```python
from build123d import *

# Parameters (mm, degrees)
SKETCH1_R           = 0.6
BOSS_EXTRUDE1_DEPTH = 6.62
SKETCH2_W           = 5.82
SKETCH2_H           = 1.74
SKETCH2_H_2         = 1.53
CUT_EXTRUDE1_DEPTH  = 14.92
SKETCH5_W           = 0.8
SKETCH5_H           = 1.53
CUT_EXTRUDE4_DEPTH  = 6.62
SKETCH4_W           = 7.64
SKETCH4_H           = 5.82
SKETCH4_W_2         = 3.88
SKETCH4_H_2         = 3.6
CUT_EXTRUDE3_DEPTH  = 7.4
CHAMFER1_SIZE       = 0.5
SKETCH11_W          = 0.34
SKETCH11_H          = 0.8
CUT_EXTRUDE5_DEPTH  = 0.9


with BuildPart() as part:
    # Sketch1 → Boss-Extrude1 (new body)
    with BuildSketch(Plane.XY):
        Polygon((3.76, 2.4), (3.76, 3.2), (11.38, 3.2), (11.38, -3.2), (3.76, -3.2), (3.76, -2.4), (-2.54, -2.4), (-2.54, 2.4), align=None)
        Circle(SKETCH1_R, mode=Mode.SUBTRACT)
    extrude(amount=BOSS_EXTRUDE1_DEPTH)

    # Sketch2 → Cut-Extrude1 (cut, through all)
    with BuildSketch(Plane(origin=(11.38, 0, 0), x_dir=(0, 0, -1), z_dir=(1, 0, 0))):
        with Locations((-2.91, 0)):
            Rectangle(SKETCH2_W, SKETCH2_H)
        with Locations((-2.91, 2.435)):
            Rectangle(SKETCH2_W, SKETCH2_H_2)
        with Locations((-2.91, -2.435)):
            Rectangle(SKETCH2_W, SKETCH2_H_2)
    extrude(amount=-CUT_EXTRUDE1_DEPTH, mode=Mode.SUBTRACT)

    # Sketch5 → Cut-Extrude4 (cut)
    with BuildSketch(Plane(origin=(11.38, 0, 0), x_dir=(0, 0, -1), z_dir=(1, 0, 0))):
        with Locations((-6.22, 2.435)):
            Rectangle(SKETCH5_W, SKETCH5_H)
        with Locations((-6.22, -2.435)):
            Rectangle(SKETCH5_W, SKETCH5_H)
    extrude(amount=-CUT_EXTRUDE4_DEPTH, mode=Mode.SUBTRACT)

    # Sketch4 → Cut-Extrude3 (cut, through all)
    with BuildSketch(Plane.XZ.offset(3.2)):
        with Locations((1.28, 2.91)):
            Rectangle(SKETCH4_W, SKETCH4_H)
        with Locations((8.24, 1.8)):
            Rectangle(SKETCH4_W_2, SKETCH4_H_2)
    extrude(amount=-CUT_EXTRUDE3_DEPTH, mode=Mode.SUBTRACT)

    # Chamfer1
    chamfer1_edges = [part.edges().sort_by_distance(p)[0] for p in [
        (-2.54, 2.4, 6.22),
        (-2.54, -2.4, 6.22),
    ]]
    chamfer(chamfer1_edges, length=CHAMFER1_SIZE)

    # Sketch11 → Cut-Extrude5 (cut)
    with BuildSketch(Plane.XZ.offset(1.67)):
        with Locations((4.93, 6.22)):
            Rectangle(SKETCH11_W, SKETCH11_H)
    cut_extrude5 = extrude(amount=-CUT_EXTRUDE5_DEPTH, mode=Mode.SUBTRACT)

    # Mirror1: Cut-Extrude5 across plane
    add(cut_extrude5.mirror(Plane.ZX), mode=Mode.SUBTRACT)


solid = part.part
```
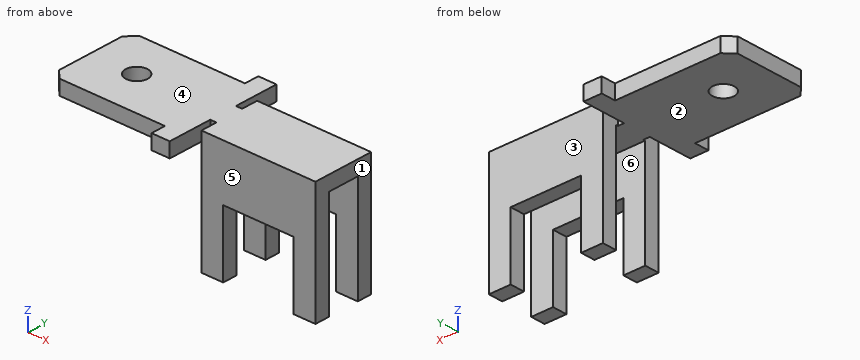
Part model, mm, in its own coordinate system. Face numbers are marked on the shaded views. A direction names the side the tool comes from. Coordinates: 2 decimals unless noted, no trailing zeros. Order: outer loops, then holes, each group sorted by start corner. A loop starts at its lowest first (then second) coordinate and runs counter-clockwise, first axis right, second up. Notation, with made-up numbers: (16.25, 48) -> (22.25, 48) arc R12 cw to (22.25, 63) -> close; hole circle Ø5 at (43, 22). An arc over 180 degrees is marked (long way). Put each result on its own line as item: value. Start each with the question number.
(1) Band-saw the part on C-C (z = 1.25). Give the cut face in (x, y).
(2) Band-saw the part on D-D (x = 10). Give the cut face in (y, z).
(3) Band-saw the part on B-B (z = 3.75). Give the cut face in (x, y).
(4) Which spindle directions (+Z, -Z, +X, -X, +Y, -Y) get a long thin tool onto all of the face, cutting with end or side? Do the marked faces 4, 5 and 6. Say none if no direction does.
(5) Mould opens along Y. For the marked faces 1, 2 and 3 say: pulls with the +Y half, pulls with the -Y half, needs draft (parallel to the pull), parting line crosses it, or undercut.
(6) Probe line 1 along X through (y, z) = (0, 6.4); line 2 along Y through (x, z) = (0, 6.35); line 3 along Z through (x, y) = (10, 1.5). List the from-to ranges inside material, lowest first. Write a range as [from, to].
(7) Band-saw the part on A-A (x = 0). Give the cut face in (y, z), then the cut area to 3 significant figures.
(8) Pin check, flat tips, straight feed: pin 1 Ø1 at (y, z) = (-1.5, 4) entering from -X; pin 2 Ø3 at (y, z) = (0.5, 4.5) entering from -X; pin 3 Ø1.5 at (y, z) = (2.5, 2.5) entering from +X; pin 4 Ø0.9 at (y, z) = (-2.5, 6) entering from +X. Stop position of each tip, or through.
Determined:
1. outline: (5.1, -1.67) -> (6.3, -1.67) -> (6.3, -0.87) -> (5.1, -0.87) -> close; (5.1, 0.87) -> (6.3, 0.87) -> (6.3, 1.67) -> (5.1, 1.67) -> close; (10.18, -1.67) -> (11.38, -1.67) -> (11.38, -0.87) -> (10.18, -0.87) -> close; (10.18, 0.87) -> (11.38, 0.87) -> (11.38, 1.67) -> (10.18, 1.67) -> close
2. outline: (-1.67, 3.6) -> (-0.87, 3.6) -> (-0.87, 5.82) -> (0.87, 5.82) -> (0.87, 3.6) -> (1.67, 3.6) -> (1.67, 6.62) -> (-1.67, 6.62) -> close
3. outline: (5.1, -1.67) -> (11.38, -1.67) -> (11.38, -0.87) -> (5.1, -0.87) -> close; (5.1, 0.87) -> (11.38, 0.87) -> (11.38, 1.67) -> (5.1, 1.67) -> close
4. face 4: +Z, +X, -X, +Y, -Y
4. face 5: +Z, -Z, +X, -Y
4. face 6: -Z, +X, -X
5. face 1: needs draft
5. face 2: undercut
5. face 3: pulls with the +Y half
6. line 1: x = [-2.54, -0.6], [0.6, 11.38]
6. line 2: y = [-2.4, -0.6], [0.6, 2.4]
6. line 3: z = [3.6, 6.62]
7. outline: (-2.4, 5.82) -> (-0.6, 5.82) -> (-0.6, 6.62) -> (-2.4, 6.62) -> close; (0.6, 5.82) -> (2.4, 5.82) -> (2.4, 6.62) -> (0.6, 6.62) -> close
7. area: 2.88 mm²
8. pin 1: stops at x = 5.1
8. pin 2: stops at x = -2.54
8. pin 3: passes through
8. pin 4: stops at x = 4.76
